Verification items for the finished model (mm, model axes). Face numbers are marked on the shaded views. A direction names the side the tool comes from. Give positions to 0.01 mm unless a question says otherwise; leave off trailing zeros. Order: outer loops, then holes, each group sorted by start corner. A loop starts at its lowest first (then second) coordinate and runs counter-clockwise, first axis right, second up.
(1) Sectioned sample at B-B on y = 12.75. Record the cut outline in (x, z), plus the area to 3 significant figures.
(2) Sectioned sample at D-D on x = 19. Record the cut outline in (y, z).
(3) Access from +Z, -Z, +X, -X, +Y, -Y to the whole of each face (thin tool, end or side, straight path). Record for the marked faces 1, 2 and 3.
(4) Gauge pin test, flat ends, axial feed: pin 1 (11 mm diameter, centred on x = 3, y = 20.5, fed in from +Z); pin 2 (16.5 mm diameter, centred on x = 21.5, y = 6.5, fed in from +Z); pin 3 (1.5 mm diameter, centred on y = 6, z = -22, fed in from -X); pin 4 (11 mm diameter, centred on x = 14.5, z = -13.5, fed in from -Y). Record the tip position at first contact, or that the pin passes through.
(5) Sectioned sample at A-A on x = 24. Record the cut outline in (y, z).
(6) Scan lines: L1, parallel to Z at x = 24, y = 13; L2, parallel to Z at x = 12.5, y = 10.75; L3, parallel to Y at x = 16, z = -11. Record each from-to range of solid material in increasing order.
(7) Sectioned sample at C-C on z = -12.75. Record the cut outline in (x, y), plus the area to 3 significant figures.
```python
from build123d import *

# Parameters (mm, degrees)
F1_DEPTH = 30
F2_DEPTH = 20
F3_DEPTH = 10
F5_DEPTH = 30.001


with BuildPart() as f1:
    # F0 (on Top) → F1 (new body)
    with BuildSketch(Plane.XY):
        Polygon((10, 15), (0, 0), (30, 0), (20, 15), align=None)
        Polygon((0, 30), (0, 0), (10, 15), align=None)
        Polygon((20, 15), (30, 0), (30, 30), align=None)
        Polygon((30, 30), (0, 30), (10, 15), (20, 15), align=None)
    extrude(amount=-F1_DEPTH)

    # F0 (on Top) → F2 (cut)
    with BuildSketch(Plane.XY):
        Polygon((10, 15), (0, 0), (30, 0), (20, 15), align=None)
    extrude(amount=-F2_DEPTH, mode=Mode.SUBTRACT)

    # F0 (on Top) → F3 (cut)
    with BuildSketch(Plane.XY):
        Polygon((0, 30), (0, 0), (10, 15), align=None)
        Polygon((20, 15), (30, 0), (30, 30), align=None)
    extrude(amount=-F3_DEPTH, mode=Mode.SUBTRACT)

    # F4 (on face) → F5 (cut, through all)
    with BuildSketch(Plane.YZ.offset(30)):
        Polygon((30, 0), (15, 0), (15, -10), align=None)
    extrude(amount=-F5_DEPTH, mode=Mode.SUBTRACT)


solid = f1.part
```
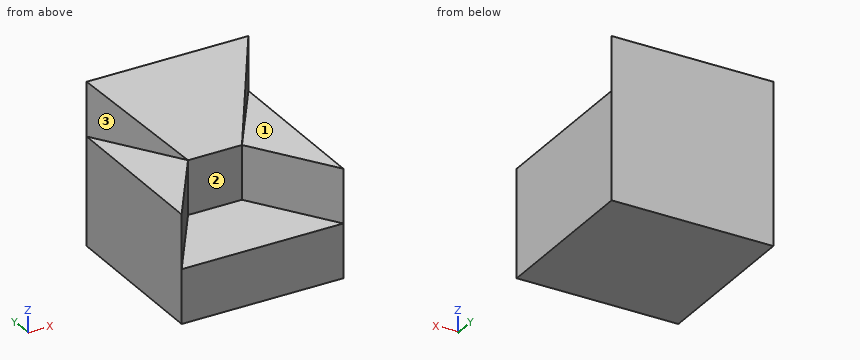
Ans:
1. outline: (0, -30) - (30, -30) - (30, -10) - (21.5, -10) - (21.5, -20) - (8.5, -20) - (8.5, -10) - (0, -10) - close
1. area: 470 mm2
2. outline: (0, -30) - (30, -30) - (30, 0) - (15, -10) - (15, -20) - (0, -20) - close
3. face 1: +Z, +X, -Y
3. face 2: +Z, -Y
3. face 3: +Z, -X, -Y
4. pin 1: stops at z = -2.67
4. pin 2: stops at z = -10
4. pin 3: stops at x = 0
4. pin 4: stops at y = 13.5
5. outline: (0, -30) - (30, -30) - (30, 0) - (21, -6) - (21, -10) - (9, -10) - (9, -20) - (0, -20) - close
6. L1: z = -30 to -10
6. L2: z = -30 to -20
6. L3: y = 15 to 30
7. outline: (0, 0) - (10, 15) - (20, 15) - (30, 0) - (30, 30) - (0, 30) - close
7. area: 600 mm2
